Source: CAD feature listing. Evaluate the final solid. Frame: model axes, mm. Face numbers are marked on the shaded views. A direction names the side the tool comes from. Give positions to 0.01 mm unless a question says otherwise; leave off trailing zeros. Loops run counter-clockwise (first coordinate to the right, second up) from the corner with the lowest first, then second, coordinate; pieces in that order, holes last. Notation, with made-up numbers: M 49.25,48.25 L 100.25,48.25 A21 ccw 100.25,83.25 Z; hole C -30.5,-40 d3. An arc over 180 degrees is marked long. Answer in a Markdown table with one row per item.
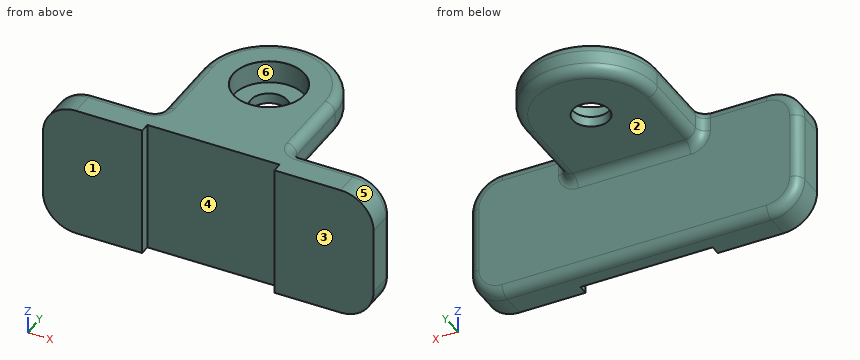
```python
from build123d import *

# Parameters (mm, degrees)
SKETCH3_W           = 100
SKETCH3_H           = 40
BOSS_EXTRUDE1_DEPTH = 10
BOSS_EXTRUDE2_DEPTH = 10
SKETCH5_W           = 40
SKETCH5_H           = 3
CUT_EXTRUDE1_DEPTH  = 85.409715081
FILLET1_R           = 10
FILLET2_R           = 3


with BuildPart() as part:
    # Sketch3 → Boss-Extrude1 (new body)
    with BuildSketch(Plane(origin=(0, 0, 0), x_dir=(1, 0, 0), z_dir=(0, 1, 0))):
        with Locations((0, 20)):
            Rectangle(SKETCH3_W, SKETCH3_H)
    extrude(amount=BOSS_EXTRUDE1_DEPTH)

    # Sketch4 → Boss-Extrude2 (add)
    with BuildSketch(Plane.XY):
        with BuildLine():
            Line((-20, 0), (-20, 35))
            ThreePointArc((-20, 35), (0, 55), (20, 35))
            Line((20, 35), (20, 0))
            Line((20, 0), (-20, 0))
        make_face()
    extrude(amount=-BOSS_EXTRUDE2_DEPTH)

    # Sketch5 → Cut-Extrude1 (cut, through all)
    with BuildSketch(Plane.XY):
        with Locations((0, 1.5)):
            Rectangle(SKETCH5_W, SKETCH5_H)
    extrude(amount=-CUT_EXTRUDE1_DEPTH, mode=Mode.SUBTRACT)

    # Sketch6 → CBORE for M10 Hex Head Bolt1 (revolve, cut)
    with BuildSketch(Plane(origin=(0, 35, 0), x_dir=(0, -1, 0), z_dir=(1, 0, 0))):
        Polygon((0, 0), (0, 40), (5.5, 40), (5.5, 6.85), (10.74, 6.85), (10.74, 0.025), (10.765, 0), align=None)
    revolve(axis=Axis((0, 35, 6.35), (0, 0, -1)), mode=Mode.SUBTRACT)

    # Fillet1
    fillet1_edges = [part.edges().sort_by_distance(p)[0] for p in [
        (-50, 5, -40),
        (50, 5, -40),
        (50, 5, 0),
        (-50, 5, 0),
    ]]
    fillet(fillet1_edges, radius=FILLET1_R)

    # Fillet2
    fillet2_edges = [part.edges().sort_by_distance(p)[0] for p in [
        (30, 10, 0),
        (-20, 22.5, -10),
        (20, 22.5, -10),
        (-20, 22.5, 0),
        (20, 22.5, 0),
        (0, 55, 0),
        (-20, 10, -5),
        (0, 55, -10),
        (20, 10, -5),
        (0, 10, -10),
        (0, 10, -40),
        (50, 10, -20),
        (-30, 10, 0),
        (-50, 10, -20),
        (-47.071067812, 10, -37.071067812),
        (-47.071067812, 10, -2.928932188),
        (47.071067812, 10, -2.928932188),
        (47.071067812, 10, -37.071067812),
    ]]
    fillet(fillet2_edges, radius=FILLET2_R)


solid = part.part
```
1) Section A-A, the plane x = 0. Return loops of the section in (y, z) (3 decimals).
Reply:
| item | result |
|---|---|
| outline | M 3,-40 L 7,-40 A3 ccw 10,-37 L 10,-13 A3 cw 13,-10 L 29.5,-10 L 29.5,-6.85 L 24.26,-6.85 L 24.26,-0.025 L 24.235,0 L 3,0 Z; M 40.5,-10 L 52,-10 A3 ccw 55,-7 L 55,-3 A3 ccw 52,0 L 45.765,0 L 45.74,-0.025 L 45.74,-6.85 L 40.5,-6.85 Z |
2) Pin query (flat end, axial travel): pin 1 Ø1 at (x, z) = (30, -24.5) entering from +Y; pin 2 Ø10.5 at (x, y) = (-1.5, 34.5) entering from +Z; pin 3 Ø10 at (y, z) = (32.5, -10.5) entering from +X. Return the tip coordinate at first contact, or that it passes through.
Reply:
| item | result |
|---|---|
| pin 1 | stops at y = 10 |
| pin 2 | stops at z = -6.85 |
| pin 3 | stops at x = 20 |
3) Set-up query: the marked faces 1 and 2. Return all of +Z, -Z, +X, -X, +Y, -Y with unobstructed straight access to the full face (end or side cutting, diameter ignored); none if empty.
Reply:
| item | result |
|---|---|
| face 1 | +Z, -Z, +X, -X, -Y |
| face 2 | -Z, +X, -X, +Y |
4) Section B-B, the plane y = 23. Return loops of the section in (x, z), then the cut area to 3 significant figures.
Reply:
| item | result |
|---|---|
| outline | M -20,-7 A3 ccw -17,-10 L 17,-10 A3 ccw 20,-7 L 20,-3 A3 ccw 17,0 L -17,0 A3 ccw -20,-3 Z |
| area | 392 mm² |
5) Material intervals for L1, parallel to Y at x = 0, z = -3; L2, parallel to Z at x = -11.5, y = 35; L3, parallel to Y at x = -45, z = -21, sorted ascending.
Reply:
| item | result |
|---|---|
| L1 | y = 3 to 24.26, 45.74 to 55 |
| L2 | z = -10 to 0 |
| L3 | y = 0 to 10 |
6) Pull-direction query (X, two-part tool) for the marked faces 3, 4, 5 and 6; classes: released by +X, released by -X, zero draft, split by the parting line, or undercut.
Reply:
| item | result |
|---|---|
| face 3 | zero draft |
| face 4 | undercut |
| face 5 | released by +X |
| face 6 | undercut |
7) Section C-C, the plane z = -16. Return loops of the section in (x, y).
Reply:
| item | result |
|---|---|
| outline | M -50,0 L -20,0 L -20,3 L 20,3 L 20,0 L 50,0 L 50,7 A3 ccw 47,10 L -47,10 A3 ccw -50,7 Z |
